```python
from build123d import *

# Parameters (mm, degrees)
SKETCH_1_W          = 78.5
SKETCH_1_H          = 53.5
EXTRUDE_1_DEPTH     = 3
SKETCH_2_W          = 2
SKETCH_2_H          = 12
CUT_EXTRUDE_1_DEPTH = 5
SKETCH_3_W          = 8
SKETCH_3_H          = 26.5
CUT_EXTRUDE_2_DEPTH = 4
SKETCH_7_W          = 2
SKETCH_7_H          = 26.5
CUT_EXTRUDE_3_DEPTH = 10
SKETCH_8_W          = 2
SKETCH_8_H          = 12
CUT_EXTRUDE_4_DEPTH = 10
SKETCH_9_W          = 2.06
SKETCH_9_H          = 12.06
SKETCH_9_W_2        = 2
SKETCH_9_H_2        = 12
CUT_EXTRUDE_5_DEPTH = 10
CHAMFER_1_SIZE      = 4
SKETCH_11_W         = 78.5
SKETCH_11_H         = 3
EXTRUDE_2_DEPTH     = 0.5
FILLET_2_R          = 2
SKETCH_14_W         = 0.08
SKETCH_14_H         = 12.06
EXTRUDE_3_DEPTH     = 3
SKETCH_15_W         = 0.08
SKETCH_15_H         = 12.06
EXTRUDE_4_DEPTH     = 3
SKETCH_16_R         = 0.5
CUT_EXTRUDE_6_DEPTH = 10
SKETCH_17_R         = 1
CUT_EXTRUDE_7_DEPTH = 10


with BuildPart() as part:
    # 草图1 → 凸台-拉伸1 (new body)
    with BuildSketch(Plane.XY):
        Rectangle(SKETCH_1_W, SKETCH_1_H)
    extrude(amount=EXTRUDE_1_DEPTH)

    # 草图2 → 切除-拉伸1 (cut)
    with BuildSketch(Plane(origin=(0, 0, 0), x_dir=(-1, 0, 0), z_dir=(0, 0, -1))):
        with Locations((-29.25, -18.25)):
            Rectangle(SKETCH_2_W, SKETCH_2_H)
    extrude(amount=-CUT_EXTRUDE_1_DEPTH, mode=Mode.SUBTRACT)

    # 草图3 → 切除-拉伸2 (cut, through all)
    with BuildSketch(Plane(origin=(0, 0, 0), x_dir=(-1, 0, 0), z_dir=(0, 0, -1))):
        with Locations((-17.625, 13.5)):
            Rectangle(SKETCH_3_W, SKETCH_3_H)
        with Locations((35.25, 13.5)):
            Rectangle(SKETCH_3_W, SKETCH_3_H)
        with Locations((17.625, 13.5)):
            Rectangle(SKETCH_3_W, SKETCH_3_H)
        with Locations((0, 13.5)):
            Rectangle(SKETCH_3_W, SKETCH_3_H)
        with Locations((-35.25, 13.5)):
            Rectangle(SKETCH_3_W, SKETCH_3_H)
    extrude(amount=-CUT_EXTRUDE_2_DEPTH, mode=Mode.SUBTRACT)

    # 草图7 → 切除-拉伸3 (cut)
    with BuildSketch(Plane(origin=(0, 0, 0), x_dir=(-1, 0, 0), z_dir=(0, 0, -1))):
        with Locations((30.25, 13.5)):
            Rectangle(SKETCH_7_W, SKETCH_7_H)
        with Locations((-30.25, 13.5)):
            Rectangle(SKETCH_7_W, SKETCH_7_H)
    extrude(amount=-CUT_EXTRUDE_3_DEPTH, mode=Mode.SUBTRACT)

    # 草图8 → 切除-拉伸4 (cut)
    with BuildSketch(Plane(origin=(0, 0, 0), x_dir=(-1, 0, 0), z_dir=(0, 0, -1))):
        with Locations((28.25, -18.25)):
            Rectangle(SKETCH_8_W, SKETCH_8_H)
    extrude(amount=-CUT_EXTRUDE_4_DEPTH, mode=Mode.SUBTRACT)

    # 草图9 → 切除-拉伸5 (cut)
    with BuildSketch(Plane(origin=(0, 0, 0), x_dir=(-1, 0, 0), z_dir=(0, 0, -1))):
        with Locations((28.25, -18.25)):
            Rectangle(SKETCH_9_W, SKETCH_9_H)
        with Locations((28.25, -18.25)):
            Rectangle(SKETCH_9_W_2, SKETCH_9_H_2, mode=Mode.SUBTRACT)
        with Locations((-29.25, -18.25)):
            Rectangle(SKETCH_9_W, SKETCH_9_H)
        with Locations((-29.25, -18.25)):
            Rectangle(SKETCH_9_W_2, SKETCH_9_H_2, mode=Mode.SUBTRACT)
    extrude(amount=-CUT_EXTRUDE_5_DEPTH, mode=Mode.SUBTRACT)

    # 倒角1
    chamfer_1_edges = [part.edges().sort_by_distance(p)[0] for p in [
        (39.25, -26.75, 1.5),
        (-39.25, -26.75, 1.5),
    ]]
    chamfer(chamfer_1_edges, length=CHAMFER_1_SIZE)

    # 草图11 → 凸台-拉伸2 (add)
    with BuildSketch(Plane(origin=(0, 0.25, 0), x_dir=(1, 0, 0), z_dir=(0, 1, 0))):
        with Locations((0, -1.5)):
            Rectangle(SKETCH_11_W, SKETCH_11_H)
    extrude(amount=EXTRUDE_2_DEPTH)

    # 圆角2
    fillet_2_edges = [part.edges().sort_by_distance(p)[0] for p in [
        (35.25, -26.75, 1.5),
        (-35.25, -26.75, 1.5),
        (-39.25, -22.75, 1.5),
        (39.25, -22.75, 1.5),
        (-39.25, 0.75, 1.5),
        (39.25, 0.75, 1.5),
    ]]
    fillet(fillet_2_edges, radius=FILLET_2_R)

    # 草图14 → 凸台-拉伸3 (add)
    with BuildSketch(Plane(origin=(0, 0, 0), x_dir=(-1, 0, 0), z_dir=(0, 0, -1))):
        with Locations((-30.24, -18.25)):
            Rectangle(SKETCH_14_W, SKETCH_14_H)
        with Locations((-28.26, -18.25)):
            Rectangle(SKETCH_14_W, SKETCH_14_H)
    extrude(amount=-EXTRUDE_3_DEPTH)

    # 草图15 → 凸台-拉伸4 (add)
    with BuildSketch(Plane(origin=(0, 0, 0), x_dir=(-1, 0, 0), z_dir=(0, 0, -1))):
        with Locations((27.26, -18.25)):
            Rectangle(SKETCH_15_W, SKETCH_15_H)
        with Locations((29.24, -18.25)):
            Rectangle(SKETCH_15_W, SKETCH_15_H)
    extrude(amount=-EXTRUDE_4_DEPTH)

    # 草图16 → 切除-拉伸6 (cut)
    with BuildSketch(Plane(origin=(0, 0, 0), x_dir=(-1, 0, 0), z_dir=(0, 0, -1))):
        with Locations((-30.2, -12.22)):
            Circle(SKETCH_16_R)
        with Locations((-28.3, -12.22)):
            Circle(SKETCH_16_R)
        with Locations((-30.2, -24.28)):
            Circle(SKETCH_16_R)
        with Locations((-28.3, -24.28)):
            Circle(SKETCH_16_R)
        with Locations((27.3, -12.22)):
            Circle(SKETCH_16_R)
        with Locations((29.2, -12.22)):
            Circle(SKETCH_16_R)
        with Locations((27.3, -24.28)):
            Circle(SKETCH_16_R)
        with Locations((29.2, -24.28)):
            Circle(SKETCH_16_R)
    extrude(amount=-CUT_EXTRUDE_6_DEPTH, mode=Mode.SUBTRACT)

    # 草图17 → 切除-拉伸7 (cut)
    with BuildSketch(Plane(origin=(0, 0, 0), x_dir=(-1, 0, 0), z_dir=(0, 0, -1))):
        with Locations((-29.25, 0.75)):
            Circle(SKETCH_17_R)
        with Locations((-21.625, 0.75)):
            Circle(SKETCH_17_R)
        with Locations((-13.625, 0.75)):
            Circle(SKETCH_17_R)
        with Locations((-4, 0.75)):
            Circle(SKETCH_17_R)
        with Locations((4, 0.75)):
            Circle(SKETCH_17_R)
        with Locations((13.625, 0.75)):
            Circle(SKETCH_17_R)
        with Locations((21.625, 0.75)):
            Circle(SKETCH_17_R)
        with Locations((29.25, 0.75)):
            Circle(SKETCH_17_R)
    extrude(amount=-CUT_EXTRUDE_7_DEPTH, mode=Mode.SUBTRACT)


solid = part.part
```
Input: part model. Units: mm. Frame: model coordinates. A direction names the side the tool comes from. Coordinates: 2 decimals unless noted, no trailing zeros. Order: outer loops, then holes, each group sorted by start corner. A loop starts at its lowest first (then second) coordinate and runs counter-clockwise, first axis right, second up. Notation, with made-up numbers: (-33, 68) - (-6, 68) arc R7 cw to (-6, 72) - close; hole circle Ø8 at (-2, -39.5). An arc over 180 degrees is marked (long way). Return JSON: item names as keys, results as strings.
Q1. Ray query, probe 1 along X at (y, z) = (9.5, 1.85) (3 decimals); probe 2 along X at (y, z) = (-18.5, 1.9). Return the intervals inside material, ascending.
The answers:
{"probe 1": "x = -29.25 to -21.625, -13.625 to -4, 4 to 13.625, 21.625 to 29.25", "probe 2": "x = -39.25 to -29.2, -27.3 to 28.3, 30.2 to 39.25"}
Q2. First-contact query: pin 1 (0.9 mm diameter, centred on x = -1, z = 1, fed in from +Y). Flat tip, straight axial feed; report the tip coordinate or a pass-through.
The answers:
{"pin 1": "stops at y = 0.75"}
Q3. Cut plane B-B (z = 1.9). State how many separate pieces and enclosed holes the cut face has, then the cut area to 3 significant figures.
The answers:
{"separate pieces": "1", "enclosed holes": "2", "area": "2,970 mm2"}
Q4. Cut plane C-C (x = 15.5). Return loops of the section in (y, z).
The answers:
{"outline": "(-26.75, 0) - (0.75, 0) - (0.75, 3) - (-26.75, 3) - close"}
Q5. Cut plane A-A (y = -19). Return loops of the section in (x, z).
The answers:
{"outline": "(-39.25, 0) - (-29.2, 0) - (-29.2, 3) - (-39.25, 3) - close; (-27.3, 0) - (28.3, 0) - (28.3, 3) - (-27.3, 3) - close; (30.2, 0) - (39.25, 0) - (39.25, 3) - (30.2, 3) - close"}
Q6. Access query for faces 1 (the flat face through (-34, 0.75, 1)), 2 (the flat face through (39.25, -12, 1)), 3 (the flat face through (-27.3, -18, 1)), 4 (the flat face through (-21.625, 14, 1)). Directions: +Z, -Z, +X, -X, +Y, -Y. A direction counts if a zero-diameter tool reaches every point of the face in a straight line with its end or side. Return the directions, or none.
The answers:
{"face 1": "+Z, -Z, -X, +Y", "face 2": "+Z, -Z, +X, +Y, -Y", "face 3": "+Z, -Z", "face 4": "+Z, -Z, +Y"}
Q7. Draft query along X for faces 5 (the flat face through (37, -25, 1)), 6 (the cylindrical face through (22.36, 0.07, 1.48)), 7 (the flat face through (0, -26.75, 1)). Return one class per face: +X half, -X half, draft (parallel to the pull), parting line (faces both ways), or undercut.
The answers:
{"face 5": "+X half", "face 6": "undercut", "face 7": "draft"}
